Answer from the drawing. Dimensions are ordinates in mm from the lowest x, y and z of the part. Coordinates: 2 decimals unless noted, no trailing zeros. Write each loop counter-clockwise with the first axis right and the second up, starting at its lowest first coordinate (ties: lowest second). Pieces come first, ordered by that corner, then holes. Notation, with made-up numbers: M 20.5,88.5 L 61.5,88.5 A9 ccw 61.5,99.5 Z; hole C 80.25,54 d6. An arc over 180 degrees is marked long. Put each result on its own line as item: value. Start each with the question number.
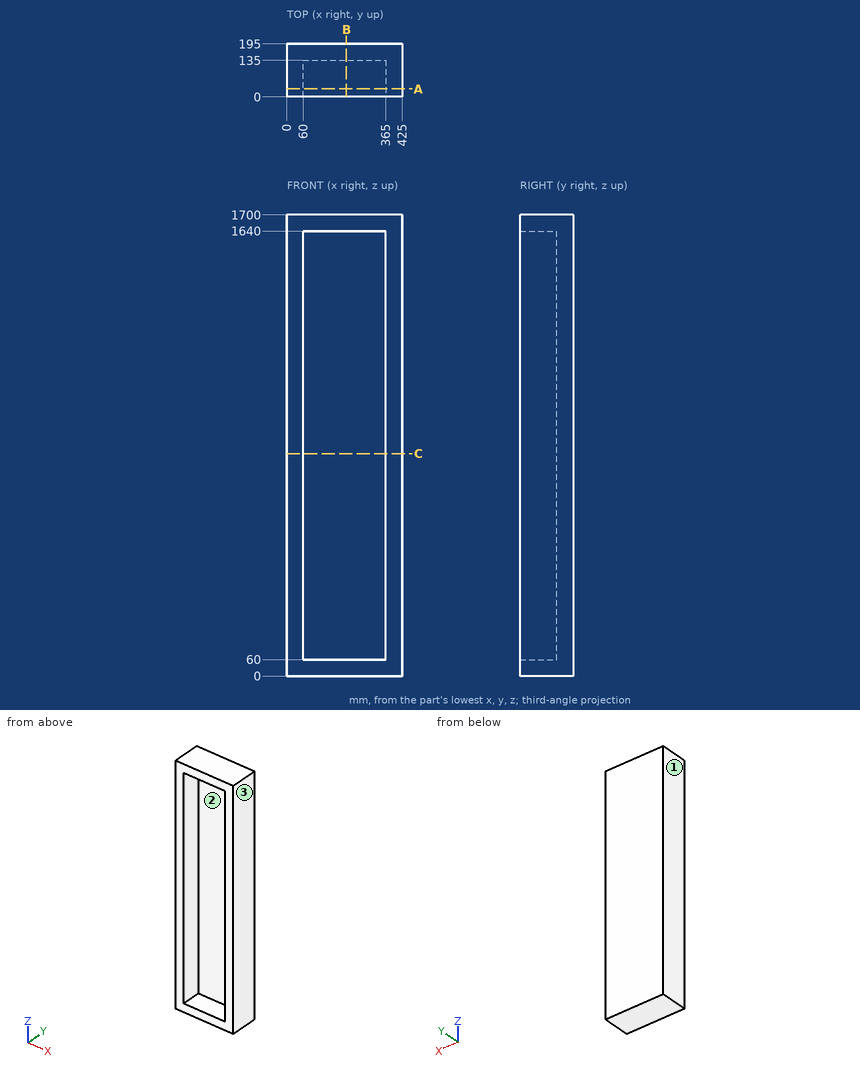
1) A cutting plane is placed at B-B on x = 219. Write down the section's boundary in (y, z).
2) Determine the mould class of the marked faces 1, 2 and 3 for opening direction X: +X half, -X half, draft (parallel to the pull), parting line (faces both ways), or undercut.
3) Straight lines are drawn through the part: probe 1 along X at (y, z) = (78.5, 901.5); probe 2 along Z at (x, y) = (65, 124); probe 3 along Y at (x, z) = (149, 867). For each, find the intervals that lie inside material, in ascending order.
4) A cutting plane is placed at A-A on y = 30. Write down the section's boundary in (x, z), then the cut area to 3 significant figures.
5) A cutting plane is placed at C-C on z = 820. Write down the section's boundary in (x, y), then the cut area to 3 significant figures.
Answers follow:
1. outline: M 0,0 L 195,0 L 195,1700 L 0,1700 L 0,1640 L 135,1640 L 135,60 L 0,60 Z
2. face 1: -X half
2. face 2: undercut
2. face 3: +X half
3. probe 1: x = 0 to 60, 365 to 425
3. probe 2: z = 0 to 60, 1640 to 1700
3. probe 3: y = 135 to 195
4. outline: M 0,0 L 425,0 L 425,1700 L 0,1700 Z; hole M 60,60 L 365,60 L 365,1640 L 60,1640 Z
4. area: 241,000 mm²
5. outline: M 0,0 L 60,0 L 60,135 L 365,135 L 365,0 L 425,0 L 425,195 L 0,195 Z
5. area: 41,700 mm²
